```python
from build123d import *

# Parameters (mm, degrees)
SKETCH_1_R               = 16
EXTRUDE_1_DEPTH          = 10
SKETCH_2_R               = 1.25
EXTRUDE_2_DEPTH          = 10.2
SKETCH_3_R               = 125
EXTRUDE_3_DEPTH          = 20
SKETCH_4_W               = 30
SKETCH_4_H               = 40
EXTRUDE_4_DEPTH          = 41.07
SKETCH_7_R               = 4.1
CUT_EXTRUDE_1_DEPTH      = 4
SKETCH_16_R              = 40
EXTRUDE_10_DEPTH         = 30
EXTRUDE_START            = -30
EXTRUDE_11_DEPTH         = 30
CUT_EXTRUDE_6_DEPTH      = 267.223590239
CUT_EXTRUDE_6_DEPTH_BACK = 267.223590239
SKETCH_18_R              = 1.25
SKETCH_19_R              = 22.5
CUT_EXTRUDE_7_DEPTH      = 180
CUT_EXTRUDE_8_DEPTH      = 217.506350946
CUT_EXTRUDE_8_DEPTH_BACK = 217.506350946
SKETCH_20_R              = 1.25
CUT_EXTRUDE_9_DEPTH      = 206.60885195
CUT_EXTRUDE_9_DEPTH_BACK = 206.60885195
SKETCH_21_R              = 2.5


with BuildPart() as part:
    # 草图1 → 凸台-拉伸1 (new body)
    with BuildSketch(Plane.XY):
        Circle(SKETCH_1_R)
    extrude(amount=EXTRUDE_1_DEPTH)

    # 草图2 → 凸台-拉伸2 (add)
    with BuildSketch(Plane(origin=(0, 0, 0), x_dir=(-1, 0, 0), z_dir=(0, 0, -1))):
        with Locations(Location((0, 12.5, 0), (0, 0, 180))):
            Circle(SKETCH_2_R)
        with Locations(Location((10.825317547, 6.25, 0), (0, 0, 180))):
            Circle(SKETCH_2_R)
        with Locations(Location((10.825317547, -6.25, 0), (0, 0, 180))):
            Circle(SKETCH_2_R)
        with Locations(Location((0, -12.5, 0), (0, 0, 180))):
            Circle(SKETCH_2_R)
        with Locations(Location((-10.825317547, -6.25, 0), (0, 0, 180))):
            Circle(SKETCH_2_R)
        with Locations(Location((-10.825317547, 6.25, 0), (0, 0, 180))):
            Circle(SKETCH_2_R)
    extrude(amount=EXTRUDE_2_DEPTH)

    # 草图3 → 凸台-拉伸3 (add)
    with BuildSketch(Plane.XY.offset(10)):
        Circle(SKETCH_3_R)
    extrude(amount=-EXTRUDE_3_DEPTH)

    # 草图4 → 凸台-拉伸4 (add)
    with BuildSketch(Plane.XY.offset(10)):
        with Locations((65, 0)):
            Rectangle(SKETCH_4_W, SKETCH_4_H)
        with Locations((-65, 0)):
            Rectangle(SKETCH_4_W, SKETCH_4_H)
    extrude(amount=EXTRUDE_4_DEPTH)

    # 草图7 → 切除-拉伸1 (cut)
    with BuildSketch(Plane(origin=(0, 0, 0), x_dir=(-1, 0, 0), z_dir=(0, 0, -1))):
        Circle(SKETCH_7_R)
    extrude(amount=-CUT_EXTRUDE_1_DEPTH, mode=Mode.SUBTRACT)

    # 草图16 → 凸台-拉伸10 (add)
    with BuildSketch(Plane.ZY.offset(80)):
        with Locations((75, 0)):
            Circle(SKETCH_16_R)
    extrude(amount=-EXTRUDE_10_DEPTH)

    # 草图17 → 凸台-拉伸11 (add)
    with BuildSketch(Plane(origin=(80, 0, 0), x_dir=(0, 0, -1), z_dir=(1, 0, 0)).offset(EXTRUDE_START)):
        with BuildLine():
            Line((-40.358983849, 20), (-51.07, 20))
            Line((-51.07, 20), (-51.07, -20))
            Line((-51.07, -20), (-40.358983849, -20))
            ThreePointArc((-40.358983849, -20), (-115, 0), (-40.358983849, 20))
        make_face()
    extrude(amount=EXTRUDE_11_DEPTH)

    # 草图18 → 切除-拉伸6 (cut, two sides: drawn at the far end of the back side and taken through both)
    with BuildSketch(Plane.ZY.offset(80).offset(-CUT_EXTRUDE_6_DEPTH_BACK)):
        with Locations((109.5, 0)):
            Circle(SKETCH_18_R)
        with Locations((106.873843872, -13.202578417)):
            Circle(SKETCH_18_R)
        with Locations((99.395183951, -24.395183951)):
            Circle(SKETCH_18_R)
        with Locations((88.202578417, -31.873843872)):
            Circle(SKETCH_18_R)
        with Locations((75, -34.5)):
            Circle(SKETCH_18_R)
        with Locations((61.797421583, -31.873843872)):
            Circle(SKETCH_18_R)
        with Locations((50.604816049, -24.395183951)):
            Circle(SKETCH_18_R)
        with Locations((43.126156128, -13.202578417)):
            Circle(SKETCH_18_R)
        with Locations((40.5, 0)):
            Circle(SKETCH_18_R)
        with Locations((43.126156128, 13.202578417)):
            Circle(SKETCH_18_R)
        with Locations((50.604816049, 24.395183951)):
            Circle(SKETCH_18_R)
        with Locations((61.797421583, 31.873843872)):
            Circle(SKETCH_18_R)
        with Locations((75, 34.5)):
            Circle(SKETCH_18_R)
        with Locations((88.202578417, 31.873843872)):
            Circle(SKETCH_18_R)
        with Locations((99.395183951, 24.395183951)):
            Circle(SKETCH_18_R)
        with Locations((106.873843872, 13.202578417)):
            Circle(SKETCH_18_R)
    extrude(amount=CUT_EXTRUDE_6_DEPTH + CUT_EXTRUDE_6_DEPTH_BACK, mode=Mode.SUBTRACT)

    # 草图19 → 切除-拉伸7 (cut)
    with BuildSketch(Plane(origin=(80, 0, 0), x_dir=(0, 0, -1), z_dir=(1, 0, 0))):
        with Locations(Location((-75, 0, 0), (0, 0, 90))):
            Circle(SKETCH_19_R)
    extrude(amount=-CUT_EXTRUDE_7_DEPTH, mode=Mode.SUBTRACT)

    # 草图20 → 切除-拉伸8 (cut, two sides: drawn at the far end of the back side and taken through both)
    with BuildSketch(Plane(origin=(0, 0, -10), x_dir=(-1, 0, 0), z_dir=(0, 0, -1)).offset(-CUT_EXTRUDE_8_DEPTH_BACK)):
        with Locations(Location((0, 12.5, 0), (0, 0, 180))):
            Circle(SKETCH_20_R)
        with Locations(Location((10.825317547, 6.25, 0), (0, 0, 180))):
            Circle(SKETCH_20_R)
        with Locations(Location((10.825317547, -6.25, 0), (0, 0, 180))):
            Circle(SKETCH_20_R)
        with Locations(Location((0, -12.5, 0), (0, 0, 180))):
            Circle(SKETCH_20_R)
        with Locations(Location((-10.825317547, -6.25, 0), (0, 0, 180))):
            Circle(SKETCH_20_R)
        with Locations(Location((-10.825317547, 6.25, 0), (0, 0, 180))):
            Circle(SKETCH_20_R)
    extrude(amount=CUT_EXTRUDE_8_DEPTH + CUT_EXTRUDE_8_DEPTH_BACK, mode=Mode.SUBTRACT)

    # 草图21 → 切除-拉伸9 (cut, two sides: drawn at the far end of the back side and taken through both)
    with BuildSketch(Plane.XY.offset(10).offset(-CUT_EXTRUDE_9_DEPTH_BACK)):
        Circle(SKETCH_21_R)
    extrude(amount=CUT_EXTRUDE_9_DEPTH + CUT_EXTRUDE_9_DEPTH_BACK, mode=Mode.SUBTRACT)


solid = part.part
```
Design review of the part built by this model. Coordinates are the model's own, in mm. A direction names the side the tool comes from. Coordinates: 2 decimals unless noted, no trailing zeros. Write each loop counter-clockwise with the first axis right and the second up, starting at its lowest first coordinate (ties: lowest second). Pieces come first, ordered by that corner, then holes.
1) To check wall thickness, follow L1, parallel to Z at x = -64.75, y = 0; L2, parallel to Y at x = 0, z = -4.25; L3, parallel to Z at x = -60.5, y = -25. State the ranges of each line that lie inside material, in increasing order.
2) Insertion check: pin 1 (3 mm diameter, centred on x = 50.5, y = -53.5, fed in from +Z); pin 2 (2 mm diameter, centred on x = -55, z = 68.5, fed in from +Y); pin 3 (3 mm diameter, centred on y = -13.2, z = 106.87, fed in from -X); pin 4 (2 mm diameter, centred on y = 34.5, z = 75, fed in from -X). Each pin has a flat end and moves straight along its axis. Give the tip position at first contact, or say it passes through.
3) Add section C-C (y = -81). Write out the cut boundary in (x, z), plus the area to 3 significant figures.
4) Add section A-A (z = 19.5). Write out the cut boundary in (x, y).
5) Add section B-B (x = 54). State how many separate pieces and enclosed holes the cut face has, plus the area to 3 significant figures.
6) Machinability: for faces 1 (the flat face through (-50, 1, 50)), 2 (the flat face through (-80, 1, 50)), 3 (the flat face through (80, 1, 50)), which of the approach directions +Z, -Z, +X, -X, +Y, -Y give a long, thin tool a straight path to every point of the face, cutting with its end or side? Answer none if there is none.
7) Mouldability with a two-part tool opening along Y and no side actions: class faces 4 (the flat face through (-65, 20, 25)), 5 (the flat face through (65, -20, 25)), 6 (the cylindrical face through (0.534, 4.065, 1.972)), 7 (the cylindrical face through (-124.88, 5.5, 0.14)) as +Y half, -Y half, draft (parallel to the pull), parting line (faces both ways), or undercut.
Check result:
1. L1: z = -10 to 39.25, 41.75 to 52.5, 97.5 to 108.25, 110.75 to 115
1. L2: y = -125 to -13.75, -11.25 to -2.5, 2.5 to 11.25, 13.75 to 125
1. L3: z = -10 to 10, 43.78 to 49.51, 51.7 to 98.3, 100.49 to 106.22
2. pin 1: stops at z = 10
2. pin 2: stops at y = 39.62
2. pin 3: stops at x = -80
2. pin 4: passes through
3. outline: (-95.21, -10) - (95.21, -10) - (95.21, 10) - (-95.21, 10) - close
3. area: 3,810 mm2
4. outline: (-80, -20) - (-50, -20) - (-50, 20) - (-80, 20) - close; (50, -20) - (80, -20) - (80, 20) - (50, 20) - close
5. separate pieces: 1
5. enclosed holes: 17
5. area: 8,940 mm2
6. face 1: +Z, +Y, -Y
6. face 2: +Z, -X, +Y, -Y
6. face 3: +Z, +X, +Y, -Y
7. face 4: +Y half
7. face 5: -Y half
7. face 6: undercut
7. face 7: parting line
